Read the model definition and answer for the solid it produces. Units are mm, in the model's axes. A direction names the side the tool comes from. Give positions to 0.01 mm unless a question says otherwise; leave off trailing zeros. Write each loop counter-clockwise with the first axis right and the second up, starting at its lowest first coordinate (ties: lowest second). Pieces come first, ordered by that corner, then holes.
```python
from build123d import *

# Parameters (mm, degrees)
F0_R      = 15
F1_DEPTH  = 12
F2_R      = 10
F3_DEPTH  = 34
F4_W      = 32.5
F4_H      = 64
F5_DEPTH  = 12
F6_R      = 16
F7_R      = 8
F8_DEPTH  = 12.001
F10_DEPTH = 4


with BuildPart() as f1:
    # F0 (on Top) → F1 (new body)
    with BuildSketch(Plane.XY):
        with BuildLine():
            Line((-22.36068, -20), (22.36068, -20))
            ThreePointArc((22.36068, -20), (0, 30), (-22.36068, -20))
        make_face()
        Circle(F0_R, mode=Mode.SUBTRACT)
    extrude(amount=-F1_DEPTH)

    # F2 (on face) → F3 (join)
    with BuildSketch(Plane(origin=(0, 0, -12), x_dir=(1, 0, 0), z_dir=(0, 0, -1))):
        with BuildLine():
            Line((15, 20), (-15, 20))
            ThreePointArc((-15, 20), (0, -25), (15, 20))
        make_face()
        Circle(F2_R, mode=Mode.SUBTRACT)
    extrude(amount=F3_DEPTH)

    # F4 (on face) → F5 (join)
    with BuildSketch(Plane(origin=(0, 0, -46), x_dir=(1, 0, 0), z_dir=(0, 0, -1))):
        with Locations((16.25, 32)):
            Rectangle(F4_W, F4_H)
        with Locations((16.25, -32)):
            Rectangle(F4_W, F4_H)
        with Locations((-16.25, 32)):
            Rectangle(F4_W, F4_H)
        with Locations((-16.25, -32)):
            Rectangle(F4_W, F4_H)
    extrude(amount=F5_DEPTH)

    # F6
    f6_edges = [f1.edges().sort_by_distance(p)[0] for p in [
        (-32.5, 64, -52),
        (32.5, 64, -52),
        (-32.5, -64, -52),
        (32.5, -64, -52),
    ]]
    fillet(f6_edges, radius=F6_R)

    # F7 (on face) → F8 (cut, through all)
    with BuildSketch(Plane.XY.offset(-46)):
        with Locations((16.5, 48)):
            Circle(F7_R)
        with Locations((-16.5, 48)):
            Circle(F7_R)
        with Locations((-16.5, -48)):
            Circle(F7_R)
        with Locations((16.5, -48)):
            Circle(F7_R)
    extrude(amount=-F8_DEPTH, mode=Mode.SUBTRACT)

    # F9 (on Right) → F10 (join, symmetric)
    with BuildSketch(Plane.YZ):
        Polygon((-20.799277, -46.774581), (-20.799277, 0), (-62.041331, -46.774581), align=None)
    extrude(amount=F10_DEPTH, both=True)


solid = f1.part
```
Item 1: Section D-D (y = 43) is taken. Write down the section's boundary in (x, z) (3 decimals).
Result set:
outline: (-32.5, -58) - (-22.745, -58) - (-22.745, -46) - (-32.5, -46) - close; (-10.255, -58) - (10.255, -58) - (10.255, -46) - (-10.255, -46) - close; (22.745, -58) - (32.5, -58) - (32.5, -46) - (22.745, -46) - close
Item 2: Section A-A (z = -51.5) is taken. Write down the section's boundary in (x, y).
Result set:
outline: (-32.5, -48) arc R16 ccw to (-16.5, -64) - (16.5, -64) arc R16 ccw to (32.5, -48) - (32.5, 48) arc R16 ccw to (16.5, 64) - (-16.5, 64) arc R16 ccw to (-32.5, 48) - close; hole circle Ø16 at (-16.5, -48); hole circle Ø16 at (-16.5, 48); hole circle Ø16 at (16.5, -48); hole circle Ø16 at (16.5, 48)
Item 3: Which of the six approach directions +Z, -Z, +X, -X, +Y, -Y give full straight-line access (tool end or side, diameter ignored) to faces 4 (the flat face through (0, 0, -46)), 5 (the flat face through (-22, 13, -46)), 6 (the flat face through (0, -20.799, -23)), 7 (the flat face through (4, -32, -33))?
Result set:
face 4: +Z
face 5: none
face 6: +Z, +X, -X
face 7: +Z, +X, -Y
Item 4: Section C-C (z = -10) is taken. Write down the section's boundary in (x, y).
Result set:
outline: (-22.36, -20) - (22.36, -20) arc R30 ccw (long way) to start; (-4, -29.62) - (4, -29.62) - (4, -20.8) - (-4, -20.8) - close; hole circle Ø30 at (0, 0)
Item 5: Determine the mould class of faces 1 (the cylindrical face through (27.937, -59.189, -52.084)), 2 (the cylindrical face through (-17.541, 55.932, -51.916)), 3 (the flat face through (-4, -32, -33)) for opening direction Y: pulls with the +Y half, pulls with the -Y half, needs draft (parallel to the pull), parting line crosses it, or undercut.
Result set:
face 1: pulls with the -Y half
face 2: undercut
face 3: needs draft
Item 6: Find the intervals of material crossed by line 1 along Y through (x, z) = (-16.5, -54.5); line 2 along X through (y, z) = (-46.5, -54); line 3 along Y through (x, z) = (0, -2), in increasing order.
Result set:
line 1: y = -64 to -56, -40 to 40, 56 to 64
line 2: x = -32.5 to -24.36, -8.64 to 8.64, 24.36 to 32.5
line 3: y = -22.56 to -20.8, -20 to -15, 15 to 30
Item 7: Each of these flat-tipped pins is pushed along its axis until it touches: pin 1 Ø4 at (x, z) = (12, -12.5) entering from -Y; pin 2 Ø5 at (x, y) = (-8, -29) entering from +Z; pin 3 Ø20.5 at (y, z) = (-33.5, -19) entering from +X. Where does it stop, or does it pass through?
Result set:
pin 1: stops at y = -20
pin 2: stops at z = -46
pin 3: stops at x = 4
Item 8: Section B-B (x = -19) is taken. Write down the section's boundary in (y, z), and give its area (3 significant figures).
Result set:
outline: (-63.8, -58) - (-55.6, -58) - (-55.6, -46) - (-63.8, -46) - close; (-40.4, -58) - (40.4, -58) - (40.4, -46) - (16.25, -46) - (16.25, -12) - (23.22, -12) - (23.22, 0) - (-20, 0) - (-20, -12) - (-16.25, -12) - (-16.25, -46) - (-40.4, -46) - close; (55.6, -58) - (63.8, -58) - (63.8, -46) - (55.6, -46) - close
area: 2,790 mm2
